Here's how the part is built. I have some questions about the finished solid (model axes, mm). A direction names the side the tool comes from. Give positions to 0.01 mm unless a question says otherwise; leave off trailing zeros. Loops run counter-clockwise (first coordinate to the right, second up) from the corner with the lowest first, then second, coordinate; pieces in that order, holes last.
Q1. For faces 5 (the face through (0.1, 7.9, 1.7)), 6 (the face through (-11, -3.25, 1)), 7 (the face through (-11, -2, 1)), 8 (the face through (11, 3.25, 1)), 9 (the face through (0, 0, 0)), which set-ups out of +Z, -Z, +X, -X, +Y, -Y let a thin tool reach every point of the face, with its end or its side?
Q2. Thinking about a two-plate mould opening in Y: for faces 1 (the face through (-11, 3.25, 1)), 2 (the face through (-15, 0, 1)), 3 (the face through (11, -3.25, 1)), 4 (the face through (12.57, -0.65, 0.51)), which applies, pulls with the +Y half, pulls with the -Y half, needs draft (parallel to the pull), parting line crosses it, or undercut?
Q3. Suppose I cut it at B-B (y = -2). List the corners of the cut face in (x, z) for me, and give its area (3 significant figures).
Q4. Suppose I cut it at A-A (z = 1.5). List the corners of the cut face in (x, y) for me.
Q5. I'm going to push flat-ended pins straight in: P1, Ø1.8, axis at x = -10, z = 2, coming from the -Y side; P2, Ø6.5, axis at x = 10.5, y = 0, coming from the +Z side; P3, Ø4.5, axis at x = 11, y = 0, coming from the +Z side. Where does each tip first touch, or does it pass through?
Q6. I need wall thicknesses on probe 1 along Y at (x, z) = (-11, 2.1); probe 2 along Y at (x, z) = (11, 0.65); probe 3 along Z at (x, y) = (-10, 1.5). Which ranges of each line are inside material? Lowest first, please.
```python
from build123d import *

# Parameters (mm, degrees)
PAD_DEPTH       = 4
SKETCH001_R     = 1.7
POCKET_DEPTH    = 4.001
SKETCH002_R     = 2.95
POCKET001_DEPTH = 3


with BuildPart() as part:
    # Sketch → Pad (new body)
    with BuildSketch(Plane.XY):
        with BuildLine():
            Line((-7.200521, 3.25), (-15, 3.25))
            Line((-15, 3.25), (-15, -3.25))
            Line((-15, -3.25), (-7.200521, -3.25))
            ThreePointArc((-7.200521, -3.25), (0, -7.9), (7.200521, -3.25))
            Line((15, -3.25), (7.200521, -3.25))
            Line((15, 3.25), (15, -3.25))
            Line((7.200521, 3.25), (15, 3.25))
            ThreePointArc((7.200521, 3.25), (0, 7.9), (-7.200521, 3.25))
        make_face()
    extrude(amount=PAD_DEPTH)

    # Sketch001 (on Face10 of Pad) → Pocket (cut, through all)
    with BuildSketch(Plane.XY.offset(4)):
        with Locations((11, 0)):
            Circle(SKETCH001_R)
        with Locations((-11, 0)):
            Circle(SKETCH001_R)
    extrude(amount=-POCKET_DEPTH, mode=Mode.SUBTRACT)

    # Sketch002 (on Face5 of Pocket) → Pocket001 (cut)
    with BuildSketch(Plane.XY.offset(4)):
        with Locations((-11, 0)):
            Circle(SKETCH002_R)
        with Locations((11, 0)):
            Circle(SKETCH002_R)
    extrude(amount=-POCKET001_DEPTH, mode=Mode.SUBTRACT)

    # Sketch003 → Groove (revolve, cut)
    with BuildSketch(Plane.YZ):
        with BuildLine():
            ThreePointArc((10, 3.083269), (5.020966, 3.770338), (0, 4))
            Line((-10, 4), (0, 4))
            Line((-10, 7), (-10, 4))
            Line((10, 7), (-10, 7))
            Line((10, 7), (10, 3.083269))
        make_face()
    revolve(axis=Axis((0, 0, -51), (0, 1, 0)), mode=Mode.SUBTRACT)


solid = part.part
```
Solutions:
1. face 5: +Z, -Z, +Y
1. face 6: +Z, -Z, -X, -Y
1. face 7: +Z
1. face 8: +Z, -Z, +X, +Y
1. face 9: -Z, +X, -X, +Y, -Y
2. face 1: pulls with the +Y half
2. face 2: needs draft
2. face 3: pulls with the -Y half
2. face 4: undercut
3. outline: (-15, 0) - (15, 0) - (15, 1.92) arc R55 ccw to (13.17, 2.4) - (13.17, 1) - (8.83, 1) - (8.83, 3.29) arc R55 ccw to (-8.83, 3.29) - (-8.83, 1) - (-13.17, 1) - (-13.17, 2.4) arc R55 ccw to (-15, 1.92) - close
3. area: 83.1 mm2
4. outline: (-15, -3.25) - (-7.2, -3.25) arc R7.9 ccw to (7.2, -3.25) - (15, -3.25) - (15, 3.25) - (7.2, 3.25) arc R7.9 ccw to (-7.2, 3.25) - (-15, 3.25) - close; hole circle Ø5.9 at (-11, 0); hole circle Ø5.9 at (11, 0)
5. P1: stops at y = -3.25
5. P2: stops at z = 3.52
5. P3: stops at z = 1
6. probe 1: y = -3.25 to -2.95, 2.95 to 3.25
6. probe 2: y = -3.25 to -1.7, 1.7 to 3.25
6. probe 3: z = 0 to 1
